from build123d import *

# Parameters (mm, degrees)
F0_W     = 350
F0_H     = 300
F1_DEPTH = 60
F2_W     = 40
F2_H     = 40
F2_W_2   = 350
F2_W_3   = 6.35
F3_DEPTH = 35


with BuildPart() as f1:
    # F0 (on Top) → F1 (new body)
    with BuildSketch(Plane.XY):
        Polygon((253.7002617121, 146.9119131565), (-216.2997382879, 146.9119131565), (-216.2997382879, 106.9119131565), (-196.2997382879, 106.9119131565), (-196.2997382879, -213.0880868435), (-216.2997382879, -213.0880868435), (-216.2997382879, -253.0880868435), (253.7002617121, -253.0880868435), (253.7002617121, -213.0880868435), (233.7002617121, -213.0880868435), (233.7002617121, 106.9119131565), (253.7002617121, 106.9119131565), align=None)
        with Locations((18.7002617121, -43.0880868435)):
            Rectangle(F0_W, F0_H, mode=Mode.SUBTRACT)
    extrude(amount=F1_DEPTH)

    # F2 (on face) → F3 (join)
    with BuildSketch(Plane.XY.offset(60)):
        with Locations((-216.2997382879, -130.2192318439)):
            Rectangle(F2_W, F2_H)
        with Locations((-176.2997382879, -130.2192318439)):
            Rectangle(F2_W, F2_H)
        with Locations((18.7002617121, -130.2192318439)):
            Rectangle(F2_W_2, F2_H)
        with Locations((213.7002617121, -130.2192318439)):
            Rectangle(F2_W, F2_H)
        with Locations((236.8752617121, -130.2192318439)):
            Rectangle(F2_W_3, F2_H)
    extrude(amount=F3_DEPTH)


solid = f1.part
Part model, mm, in its own coordinate system. A direction names the side the tool comes from. Give positions to 0.01 mm unless a question says otherwise; leave off trailing zeros. Write each loop counter-clockwise with the first axis right and the second up, starting at its lowest first coordinate (ties: lowest second). Pieces come first, ordered by that corner, then holes.
1) Cut at C-C on y = 67.5. Write the cut outline in (x, z), then the cut area to 3 significant figures.
Resolved:
outline: (-196.3, 0) - (-156.3, 0) - (-156.3, 60) - (-196.3, 60) - close; (193.7, 0) - (233.7, 0) - (233.7, 60) - (193.7, 60) - close
area: 4,800 mm2
2) Which spindle directions (+Z, -Z, +X, -X, +Y, -Y) get a long thin tool onto all of the face, cutting with end or side? Do faces 4 (the face through (244, -213.088, 30)), 5 (the face through (-206, -213.088, 30)), 6 (the face through (-156.3, -45, 30)). Say none if no direction does.
Resolved:
face 4: +Z, -Z, +X
face 5: +Z, -Z, -X
face 6: -Z
3) Two-plate mould, pull along Y, no slides. Class faces 1 (the face through (253.7, -233, 30)), 2 (the face through (-217, -130, 60)), 3 (the face through (5, -110.219, 77)): released by +Y, released by -Y, zero draft, split by the parting line, or undercut.
Resolved:
face 1: zero draft
face 2: undercut
face 3: released by +Y
4) Pin check, flat tips, straight feed: pin 1 (18 mm diameter, centred on y = -24, z = 23, fed in from +X); pin 2 (3 mm diameter, centred on y = -104, z = 22.5, fed in from -X); pin 3 (6 mm diameter, centred on x = -178.5, z = 77, fed in from -Y). Stop position of each tip, or through.
Resolved:
pin 1: stops at x = 233.7
pin 2: stops at x = -196.3
pin 3: stops at y = -150.22
5) Cut at A-A on z = 14. Write the cut outline in (x, y).
Resolved:
outline: (-216.3, -253.09) - (253.7, -253.09) - (253.7, -213.09) - (233.7, -213.09) - (233.7, 106.91) - (253.7, 106.91) - (253.7, 146.91) - (-216.3, 146.91) - (-216.3, 106.91) - (-196.3, 106.91) - (-196.3, -213.09) - (-216.3, -213.09) - close; hole (-156.3, -193.09) - (193.7, -193.09) - (193.7, 106.91) - (-156.3, 106.91) - close
6) Cut at B-B on x = 79. Write the cut outline in (y, z), then the cut area to 3 significant figures.
Resolved:
outline: (-253.09, 0) - (-193.09, 0) - (-193.09, 60) - (-253.09, 60) - close; (-150.22, 60) - (-110.22, 60) - (-110.22, 95) - (-150.22, 95) - close; (106.91, 0) - (146.91, 0) - (146.91, 60) - (106.91, 60) - close
area: 7,400 mm2
7) Cut at D-D on y = -128.5. Write the cut outline in (x, z), then the cut area to 3 significant figures.
Resolved:
outline: (-236.3, 60) - (-196.3, 60) - (-196.3, 0) - (-156.3, 0) - (-156.3, 60) - (193.7, 60) - (193.7, 0) - (233.7, 0) - (233.7, 60) - (240.05, 60) - (240.05, 95) - (-236.3, 95) - close
area: 21,500 mm2
8) Probe L1, parallel to Y at x = 29, z = 41; L2, parallel to X at y = -74, z = 5.5; L3, parallel to Z at x = 96, y = -122.5. List the from-to ranges inside material, lowest first.
Resolved:
L1: y = -253.09 to -193.09, 106.91 to 146.91
L2: x = -196.3 to -156.3, 193.7 to 233.7
L3: z = 60 to 95
